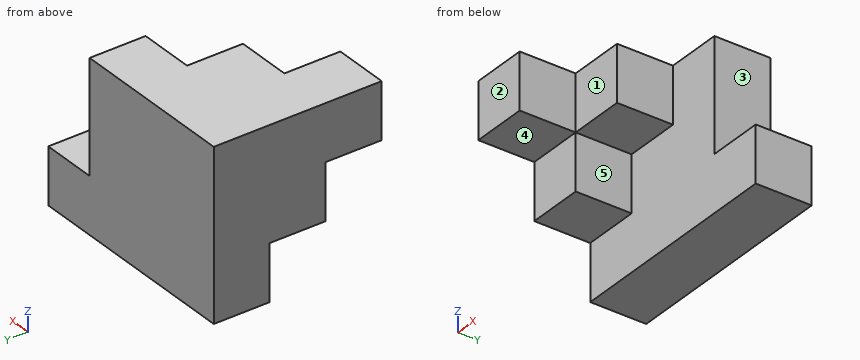
```python
from build123d import *

# Parameters (mm, degrees)
F0_W     = 101.6
F0_H     = 76.2
F1_DEPTH = 25.4
F2_W     = 25.4
F2_H     = 50.8
F3_DEPTH = 25.4
F4_W     = 50.8
F4_H     = 50.8
F5_DEPTH = 25.4
F6_W     = 25.4
F6_H     = 25.4
F7_DEPTH = 25.4
F8_W     = 25.4
F8_H     = 25.4
F9_DEPTH = 25.4


with BuildPart() as f1:
    # F0 (on Front) → F1 (new body)
    with BuildSketch(Plane.XZ):
        with Locations((50.8, 38.1)):
            Rectangle(F0_W, F0_H)
    extrude(amount=F1_DEPTH)

    # F2 (on face) → F3 (cut)
    with BuildSketch(Plane.XZ.offset(25.4)):
        with Locations((88.9, 50.8)):
            Rectangle(F2_W, F2_H)
    extrude(amount=-F3_DEPTH, mode=Mode.SUBTRACT)

    # F4 (on face) → F5 (join)
    with BuildSketch(Plane.XZ.offset(25.4)):
        with Locations((25.4, 50.8)):
            Rectangle(F4_W, F4_H)
    extrude(amount=F5_DEPTH)

    # F6 (on face) → F7 (cut)
    with BuildSketch(Plane.XZ.offset(50.8)):
        with Locations((38.1, 38.1)):
            Rectangle(F6_W, F6_H)
    extrude(amount=-F7_DEPTH, mode=Mode.SUBTRACT)

    # F8 (on face) → F9 (join)
    with BuildSketch(Plane.XZ.offset(50.8)):
        with Locations((12.7, 63.5)):
            Rectangle(F8_W, F8_H)
    extrude(amount=F9_DEPTH)


solid = f1.part
```
Geometry: final body of the model. Coordinates: model frame, mm. Face numbers are marked on the shaded views. A direction names the side the tool comes from. Give positions to 0.01 mm unless a question says otherwise; leave off trailing zeros. Order: outer loops, then holes, each group sorted by start corner. A loop starts at its lowest first (then second) coordinate and runs counter-clockwise, first axis right, second up. Notation, with made-up numbers: (32, 88.25) -> (79, 88.25) arc R23 cw to (79, 108.25) -> close; hole circle Ø8 at (-0.5, -33). An arc over 180 degrees is marked (long way). Write each question's results on one line, items separated by ' | '. Start each with the question number.
1) Section D-D (y = -27). Return loops of the section in (x, z), then the cut area to 3 significant figures.
2) Section A-A (y = -14). Return loops of the section in (x, z).
3) Section C-C (x = 21). Return loops of the section in (y, z).
4) Section B-B (z = 70). Return loops of the section in (x, y).
5) Line query: line 1 (X direction, y = -34.5, z = 34); line 2 (X direction, y = -41.5, z = 51.5). Output: solid intervals per line, ascending. Write a range as from..to.
6) Set-up query: the marked faces 1, 2, 3, 4 and 5. Return all of +Z, -Z, +X, -X, +Y, -Y with unobstructed straight access to the full face (end or side cutting, diameter ignored); none if empty.
7) First-contact query: pin 1 (7.5 mm diameter, centred on y = -44.5, z = 38.5, fed in from +X); pin 2 (7.5 mm diameter, centred on y = -8.5, z = 58.5, fed in from +X); pin 3 (20.5 mm diameter, centred on x = 92.5, y = -10.5, fed in from +Z). Flat tips, straight axial feed; report the tip coordinate or a pass-through.
Calculated:
1) outline: (0, 25.4) -> (25.4, 25.4) -> (25.4, 50.8) -> (50.8, 50.8) -> (50.8, 76.2) -> (0, 76.2) -> close | area: 1,940 mm2
2) outline: (0, 0) -> (101.6, 0) -> (101.6, 25.4) -> (76.2, 25.4) -> (76.2, 76.2) -> (0, 76.2) -> close
3) outline: (-76.2, 50.8) -> (-50.8, 50.8) -> (-50.8, 25.4) -> (-25.4, 25.4) -> (-25.4, 0) -> (0, 0) -> (0, 76.2) -> (-76.2, 76.2) -> close
4) outline: (0, -76.2) -> (25.4, -76.2) -> (25.4, -50.8) -> (50.8, -50.8) -> (50.8, -25.4) -> (76.2, -25.4) -> (76.2, 0) -> (0, 0) -> close
5) line 1: 0..25.4 | line 2: 0..50.8
6) face 1: +Z, -Z, +X, -Y | face 2: +Z, -Z, +X, -X, -Y | face 3: +Z, +X, +Y, -Y | face 4: -Z, +X, -X, -Y | face 5: -Z, +X, -Y
7) pin 1: x = 25.4 | pin 2: x = 76.2 | pin 3: z = 25.4
